Part model, mm, in its own coordinate system. A direction names the side the tool comes from. Give positions to 0.01 mm unless a question says otherwise; leave off trailing zeros. Write each loop counter-clockwise with the first axis right and the second up, starting at its lowest first coordinate (ties: lowest second). Pieces come first, ordered by that corner, then holes. Notation, with made-up numbers: M 46.25,-30 L 51.25,-30 A14 ccw 51.25,-6 Z; hole C 80.5,50 d3. An arc over 180 degrees is marked long. Use CSV: the item, a comma, the result in double quotes. Start each with the question number.
Item 1: Cut at D-D (x = 1.5). List the corners of the cut face in (y, z).
Item 2: Which spindle directions (+Z, -Z, +X, -X, +Y, -Y) get a long thin tool onto all of the face, cutting with end or side? Do faces 1 (the flat face through (32.085, 44.368, 0.229)), 2 (the flat face through (31.604, 42.275, -0.493)), 3 (the flat face through (-31.44, 42.35, -0.49)). Say none if no direction does.
Item 3: Drill centre lines: line 1 (Z direction, x = -39, y = 37.5); line 2 (X direction, y = -22, z = -16). Where is each one in solid material? Low to high. Write a range as [from, to].
Item 4: Cut at C-C (z = -32). List the corners of the cut face in (x, y).
Item 5: Pin check, flat tips, straight feed: pin 1 (6 mm diameter, centred on y = 19, z = -31.5, fed in from -X); pin 2 (3.5 mm diameter, centred on x = 46.07, y = -20.13, fed in from +Z); pin 3 (1.1 mm diameter, centred on x = 45.5, z = -0.5, fed in from +Y); pin 4 (1.1 mm diameter, centred on x = 50.5, z = -17, fed in from +Y). Stop position of each tip, or through.
Item 6: Cut at A-A (x = -41). List the corners of the cut face in (y, z), then the cut area to 3 significant figures.
Item 7: Cut at B-B (y = 17.5). List the corners of the cut face in (x, z).
Item 8: Mould opens along X. For faces 4 (the flat face through (49.726, 5, -20)), 5 (the cylindrical face through (-46.483, 29.849, 0.521)), 6 (the cylindrical face through (31.86, 44.34, 0.94)), 7 (the cylindrical face through (-46.53, -20.71, 0.52)) say: released by +X, released by -X, zero draft, split by the parting line, or undercut.
Autodesk Inventor part; units mm, degrees
ref_plane "YZ Plane" through (0, 0, 0) normal (1, 0, 0) x (0, 1, 0)
ref_plane "XZ Plane" through (0, 0, 0) normal (0, 1, 0) x (-1, 0, 0)
ref_plane "XY Plane" through (0, 0, 0) normal (0, 0, 1) x (1, 0, 0)
sketch "Sketch1" plane through (0, 0, 0) normal (0, 0, 1) x (1, 0, 0)
  line L0 (25.0566, 47.4388) -> (-25.0566, 47.4388)
  line L1 (-25.9018, 47.2514) -> (-38.0982, 41.5642)
  line L2 (-38.9434, 41.3768) -> (-53.924, 41.3768)
  line L3 (-55.924, 39.3768) -> (-55.924, -30.1412)
  line L4 (-53.924, -32.1412) -> (62.994, -32.1412)
  line L5 (64.994, -30.1412) -> (64.994, 39.3768)
  line L6 (62.994, 41.3768) -> (38.9434, 41.3768)
  line L7 (38.0982, 41.5642) -> (25.9018, 47.2514)
  line L8 (0, 0) -> (0, 61.2972) construction
  arc A0 (64.994, 39.3768) -> (62.994, 41.3768) centre (62.994, 39.3768) ccw
  arc A1 (62.994, -32.1412) -> (64.994, -30.1412) centre (62.994, -30.1412) ccw
  arc A2 (-55.924, -30.1412) -> (-53.924, -32.1412) centre (-53.924, -30.1412) ccw
  arc A3 (-53.924, 41.3768) -> (-55.924, 39.3768) centre (-53.924, 39.3768) ccw
  arc A4 (-38.9434, 41.3768) -> (-38.0982, 41.5642) centre (-38.9434, 43.3768) ccw
  arc A5 (-25.0566, 47.4388) -> (-25.9018, 47.2514) centre (-25.0566, 45.4388) ccw
  arc A6 (25.9018, 47.2514) -> (25.0566, 47.4388) centre (25.0566, 45.4388) ccw
  arc A7 (38.0982, 41.5642) -> (38.9434, 41.3768) centre (38.9434, 43.3768) ccw
  point P0 (25.5, 47.4388)
  point P1 (-25.5, 47.4388)
  point P2 (-38.5, 41.3768)
  point P3 (-55.924, 41.3768)
  point P4 (-55.924, -32.1412)
  point P5 (64.994, 41.3768)
  point P6 (38.5, 41.3768)
  point P7 (0, 47.4388)
  dimension "d48" = 51
  dimension "d50" = 155
  dimension "d51" = 155
  dimension "d52" = 13
  dimension "d53" = 17.424
  dimension "d54" = 26.494
  dimension "d55" = 73.518
  dimension "d56" = 13
  dimension "d57" = 2
extrude "Extrusion1" add sketch "Sketch1" along normal blind 2
chamfer "Chamfer1" distance 1.5 distance2 1 16 edges at (50.9687, 41.3768, 2) (38.5105, 41.4242, 2) (32, 44.4078, 2) (25.4895, 47.3914, 2) (0, 47.4388, 2) (-25.4895, 47.3914, 2) (-32, 44.4078, 2) (-38.5105, 41.4242, 2) (-46.4337, 41.3768, 2) (-55.3382, 40.791, 2) (-55.924, 4.6178, 2) (-55.3382, -31.5554, 2) (4.535, -32.1412, 2) (64.4082, -31.5554, 2) (64.994, 4.6178, 2) (64.4082, 40.791, 2) measured on face at (11.3755, -5.6145, 2)
fillet "Fillet1" radius 2 16 edges at (-54.2776, 39.7304, 2) (-46.4337, 39.8768, 2) (-38.1859, 39.9598, 2) (-31.3661, 43.0484, 2) (-25.1648, 45.927, 2) (0, 45.9388, 2) (25.1648, 45.927, 2) (31.3661, 43.0484, 2) (38.1859, 39.9598, 2) (50.9687, 39.8768, 2) (63.3476, 39.7304, 2) (63.494, 4.6178, 2) (63.3476, -30.4947, 2) (4.535, -30.6412, 2) (-54.2776, -30.4947, 2) (-54.424, 4.6178, 2)
fillet "Fillet2" radius 1 16 edges at (-55.3382, -31.5554, 1) (4.535, -32.1412, 1) (64.4082, -31.5554, 1) (64.994, 4.6178, 1) (64.4082, 40.791, 1) (50.9687, 41.3768, 1) (38.5105, 41.4242, 1) (32, 44.4078, 1) (25.4895, 47.3914, 1) (0, 47.4388, 1) (-25.4895, 47.3914, 1) (-32, 44.4078, 1) (-38.5105, 41.4242, 1) (-46.4337, 41.3768, 1) (-55.3382, 40.791, 1) (-55.924, 4.6178, 1)
feature "Lip1" [suppressed]
sketch "Sketch8" plane through (0, 0, 0) normal (0, 0, -1) x (-1, 0, 0)
  line L0 (-64.994, 39.3768) -> (-64.994, -30.1412)
  arc A0 (-64.994, -30.1412) -> (-62.994, -32.1412) centre (-62.994, -30.1412) ccw
  line L1 (-62.994, -32.1412) -> (53.924, -32.1412)
  arc A1 (53.924, -32.1412) -> (55.924, -30.1412) centre (53.924, -30.1412) ccw
  line L2 (55.924, -30.1412) -> (55.924, 39.3768)
  arc A2 (55.924, 39.3768) -> (53.924, 41.3768) centre (53.924, 39.3768) ccw
  line L3 (53.924, 41.3768) -> (38.9434, 41.3768)
  arc A3 (38.0982, 41.5642) -> (38.9434, 41.3768) centre (38.9434, 43.3768) ccw
  line L4 (38.0982, 41.5642) -> (25.9018, 47.2514)
  arc A4 (25.9018, 47.2514) -> (25.0566, 47.4388) centre (25.0566, 45.4388) ccw
  line L5 (25.0566, 47.4388) -> (-25.0566, 47.4388)
  arc A5 (-25.0566, 47.4388) -> (-25.9018, 47.2514) centre (-25.0566, 45.4388) ccw
  line L6 (-25.9018, 47.2514) -> (-38.0982, 41.5642)
  arc A6 (-38.9434, 41.3768) -> (-38.0982, 41.5642) centre (-38.9434, 43.3768) ccw
  line L7 (-38.9434, 41.3768) -> (-62.994, 41.3768)
  arc A7 (-62.994, 41.3768) -> (-64.994, 39.3768) centre (-62.994, 39.3768) ccw
  line L8 (-60.894, 39.2768) -> (-38.9434, 39.2768)
  arc A8 (-38.9434, 39.2768) -> (-37.2107, 39.661) centre (-38.9434, 43.3768) ccw
  line L9 (-37.2107, 39.661) -> (-25.8381, 44.964)
  line L10 (-24.1477, 45.3388) -> (24.1477, 45.3388)
  line L11 (25.8381, 44.964) -> (37.2107, 39.661)
  arc A9 (37.2107, 39.661) -> (38.9434, 39.2768) centre (38.9434, 43.3768) ccw
  line L12 (38.9434, 39.2768) -> (51.824, 39.2768)
  line L13 (53.824, 37.2768) -> (53.824, -28.0412)
  line L14 (51.824, -30.0412) -> (-60.894, -30.0412)
  line L15 (-62.894, -28.0412) -> (-62.894, 37.2768)
  arc A10 (-60.894, 39.2768) -> (-62.894, 37.2768) centre (-60.894, 37.2768) ccw
  arc A11 (-62.894, -28.0412) -> (-60.894, -30.0412) centre (-60.894, -28.0412) ccw
  arc A12 (51.824, -30.0412) -> (53.824, -28.0412) centre (51.824, -28.0412) ccw
  arc A13 (53.824, 37.2768) -> (51.824, 39.2768) centre (51.824, 37.2768) ccw
  arc A14 (-24.1477, 45.3388) -> (-25.8381, 44.964) centre (-24.1477, 41.3388) ccw
  arc A15 (25.8381, 44.964) -> (24.1477, 45.3388) centre (24.1477, 41.3388) ccw
  point P0 (0, 0)
  dimension "d62" = 2.1
  dimension "d63" = 2
  dimension "d64" = 4
extrude "Extrusion7" add sketch "Sketch8" along normal blind 1 contours L8 A8 L9 A14 L10 A15 L11 A9 L12 A13 L13 A12 L14 A11 L15 A10
sketch "Sketch4" plane through (0, 0, 2) normal (0, 0, 1) x (1, 0, 0)
  line L0 (92.6097, 61.0907) -> (51.0597, 61.0907)
  line L1 (51.0597, 61.0907) -> (51.0597, -62.6292)
  line L2 (51.0597, -62.6292) -> (92.6097, -62.6292)
  line L3 (92.6097, -62.6292) -> (92.6097, 61.0907)
  line L4 (64.5487, 39.3768) -> (64.5487, -30.1412)
  point P0 (0, 0)
  dimension "d21" = 123.7199
  dimension "d22" = 41.55
  dimension "d58" = 13.489
extrude "Extrusion3" cut sketch "Sketch4" against normal blind 10
sketch "Sketch7" plane through (0, 0, 0) normal (0, 0, -1) x (-1, 0, 0)
  line L0 (-51.0597, 38.2572) -> (-49.7257, 38.2572)
  line L1 (-49.7257, 38.2572) -> (-49.7257, -29.0608)
  line L2 (-49.7257, -29.0608) -> (-51.0597, -29.0608)
  line L3 (-51.0597, -29.0608) -> (-51.0597, 38.2572)
  line L4 (-51.0597, -30.0412) -> (-51.0597, -32.1412)
  line L5 (53.924, -30.8108) -> (-51.0597, -30.8108)
  line L6 (-51.0597, 42.7072) -> (-38.8527, 42.7072)
  point P0 (0, 0)
  point P1 (-51.0597, -28.8108)
  point P2 (-51.0597, 40.7072)
  point P3 (-32.4217, 42.6092)
  dimension "d35" = 1.334
  dimension "d59" = 1.75
  dimension "d60" = 4.45
  dimension "d61" = 67.318
extrude "Extrusion6" add sketch "Sketch7" along normal blind 39
sketch "Sketch9" plane through (0, 0, 2) normal (0, 0, 1) x (1, 0, 0)
  circle A0 centre (-47.914, 29.3988) radius 1.5
  circle A1 centre (-47.914, -20.1312) radius 1.5
  circle A2 centre (46.066, 29.3988) radius 1.5
  circle A3 centre (46.066, -20.1312) radius 1.5
  point P0 (0, 0)
extrude "Extrusion8" cut sketch "Sketch9" against normal blind 10
properties part number "Simple3DPrintBackplate01" material "Aluminum 6061 Black Anodized"
Worked answers:
1,outline,"M -32.14,0 L -30.04,0 L -30.04,-1 L 45.34,-1 L 45.34,0 L 47.44,0 L 47.44,0.46 A1 ccw 46.99,1.3 L 46.44,1.66 A2 ccw 45.33,2 L -30.04,2 A2 ccw -31.15,1.66 L -31.7,1.3 A1 ccw -32.14,0.46 Z"
2,face 1,"+Z, -Z, +X, +Y"
2,face 2,"-Z, +X, +Y"
2,face 3,"-Z, -X, +Y"
3,line 1,"z = [-1, 2]"
3,line 2,"x = [49.73, 51.06]"
4,outline,"M 49.73,-29.06 L 51.06,-29.06 L 51.06,38.26 L 49.73,38.26 Z"
5,pin 1,"stops at x = 49.73"
5,pin 2,"stops at z = 2"
5,pin 3,"stops at y = 41.38"
5,pin 4,"stops at y = 38.26"
6,outline,"M -32.14,0 L -30.04,0 L -30.04,-1 L 39.28,-1 L 39.28,0 L 41.38,0 L 41.38,0.46 A1 ccw 40.93,1.3 L 40.38,1.66 A2 ccw 39.27,2 L -30.04,2 A2 ccw -31.15,1.66 L -31.7,1.3 A1 ccw -32.14,0.46 Z"
6,area,"215 mm^2"
7,outline,"M -55.92,0 L -53.82,0 L -53.82,-1 L 49.73,-1 L 49.73,-39 L 51.06,-39 L 51.06,2 L -53.82,2 A2 ccw -54.93,1.66 L -55.48,1.3 A1 ccw -55.92,0.46 Z"
8,face 4,"released by -X"
8,face 5,"undercut"
8,face 6,"released by +X"
8,face 7,"undercut"
